from build123d import *

# Parameters (mm, degrees)
F0_R     = 11
F1_DEPTH = 2
F2_R     = 2.99
F3_DEPTH = 8.5
F4_R     = 0.2


with BuildPart() as f1:
    # F0 (on Top) → F1 (new body)
    with BuildSketch(Plane.XY):
        Circle(F0_R)
    extrude(amount=F1_DEPTH)

    # F2 (on face) → F3 (join)
    with BuildSketch(Plane.XY.offset(2)):
        Circle(F2_R)
    extrude(amount=F3_DEPTH)

    # F4
    f4_edges = [f1.edges().sort_by_distance(p)[0] for p in [
        (-11, 0, 2),
        (-11, 0, 0),
        (-2.99, 0, 10.5),
    ]]
    fillet(f4_edges, radius=F4_R)


solid = f1.part
Verification items for the finished model (mm, model axes). A direction names the side the tool comes from. Give positions to 0.01 mm unless a question says otherwise; leave off trailing zeros. Loops run counter-clockwise (first coordinate to the right, second up) from the corner with the lowest first, then second, coordinate; pieces in that order, holes last.
1. Cross-section at B-B on z = 3.75. Record the cut outline in (x, y).
Derived:
outline: circle Ø5.98 at (0, 0)
2. Cross-section at A-A on x = 0. Record the cut outline in (y, z), and give its area (3 significant figures).
Derived:
outline: (-11, 0.2) arc R0.2 ccw to (-10.8, 0) - (10.8, 0) arc R0.2 ccw to (11, 0.2) - (11, 1.8) arc R0.2 ccw to (10.8, 2) - (2.99, 2) - (2.99, 10.3) arc R0.2 ccw to (2.79, 10.5) - (-2.79, 10.5) arc R0.2 ccw to (-2.99, 10.3) - (-2.99, 2) - (-10.8, 2) arc R0.2 ccw to (-11, 1.8) - close
area: 94.8 mm2
3. Material ranges on probe 1 along Z at (x, y) = (-2.75, -6.75); probe 2 along Y at (x, z) = (0, 5); probe 3 along Y at (x, z) = (-6.5, 1), recorded low to high.
Derived:
probe 1: z = 0 to 2
probe 2: y = -2.99 to 2.99
probe 3: y = -8.87 to 8.87
4. Go/stop test with flat-tipped pins: P1, Ø1, axis at x = -0.5, z = 9.5, coming from the +Y side; P2, Ø11, axis at x = 1.5, y = 3.5, coming from the +Z side; P3, Ø1, axis at x = -3, z = 6, coming from the -Y side; P4, Ø1.5, axis at y = -1.5, z = 3.5, coming from the +X side. Record where each tip stops, or that it passes through.
Derived:
P1: stops at y = 2.99
P2: stops at z = 10.5
P3: stops at y = -1.64
P4: stops at x = 2.89
5. Tool access check on faces 1 (the flat face through (0, 0, 0)), 2 (the flat face through (2.25, -2.25, 2)). Record the directions out of +Z, -Z, +X, -X, +Y, -Y that give a thin tool (end or side, any length) a straight path to the whole face; none if there is none.
Derived:
face 1: -Z, +X, -X, +Y, -Y
face 2: +Z
